Autodesk Inventor part; units mm, degrees
ref_plane "YZ Plane" through (0, 0, 0) normal (1, 0, 0) x (0, 1, 0)
ref_plane "XZ Plane" through (0, 0, 0) normal (0, 1, 0) x (-1, 0, 0)
ref_plane "XY Plane" through (0, 0, 0) normal (0, 0, 1) x (1, 0, 0)
sketch "Sketch1" plane through (0, 0, 0) normal (0, 0, 1) x (1, 0, 0)
  line L0 (0, 0) -> (28.575, 0)
  line L1 (28.575, 0) -> (28.575, 19.05)
  line L2 (28.575, 19.05) -> (0, 19.05)
  line L3 (0, 19.05) -> (0, 0)
  arc A0 (23.8125, 14.2875) -> (23.8125, 7.9375) centre (23.8125, 11.1125) ccw
  arc A1 (4.7625, 7.9375) -> (4.7625, 14.2875) centre (4.7625, 11.1125) ccw
  line L4 (0, 7.9375) -> (4.7625, 7.9375)
  line L5 (0, 14.2875) -> (4.7625, 14.2875)
  line L6 (28.575, 14.2875) -> (23.8125, 14.2875)
  line L7 (28.575, 7.9375) -> (23.8125, 7.9375)
  dimension "d4" = 28.575
  dimension "d5" = 19.05
  dimension "d18" = 7.9375
  dimension "d19" = 4.7625
  dimension "d20" = 7.9375
  dimension "d21" = 4.7625
  dimension "d22" = 6.35
  dimension "d23" = 6.35
  dimension "d24" = 4.7625
  dimension "d25" = 4.7625
  dimension "d26" = 4.7625
  dimension "d27" = 4.7625
extrude "Extrusion1" add sketch "Sketch1" along normal blind 3.175
sketch "Sketch3" plane through (0, 19.05, 0) normal (0, 1, 0) x (1, 0, 0)
  line L0 (0, 0) -> (28.575, 0)
  line L1 (0, 0) -> (28.575, 0)
  line L2 (28.575, 0) -> (28.575, -6.35)
  line L3 (28.575, -6.35) -> (0, -6.35)
  line L4 (0, 0) -> (0, -3.175)
  line L5 (0, 0) -> (0, -22.225)
  circle A0 centre (6.35, -22.225) radius 6.35
  line L6 (28.575, -6.35) -> (11.1411, -26.3925)
  circle A1 centre (6.35, -22.225) radius 3.175
  dimension "d6" = 6.35
  dimension "d8" = 22.225
  dimension "d10" = 28.575
  dimension "d12" = 12.7
  dimension "d13" = 6.35
  dimension "d16" = 6.35
extrude "Extrusion2" add sketch "Sketch3" along normal blind 3.175
fillet "Fillet1" radius 3.175 1 edges at (14.2875, 22.225, 0)
sketch "Sketch4" plane through (0, 0, 0) normal (0, 0, -1) x (-1, 0, 0)
  arc A0 (-23.8125, 7.9375) -> (-23.8125, 14.2875) centre (-23.8125, 11.1125) ccw
  arc A1 (-4.7625, 14.2875) -> (-4.7625, 7.9375) centre (-4.7625, 11.1125) ccw
  line L0 (-28.575, 19.05) -> (0, 19.05)
  line L1 (-28.575, 0) -> (-28.575, 19.05)
  line L2 (0, 0) -> (0, 19.05)
  line L3 (-28.575, 0) -> (-28.575, 19.05)
  line L4 (-28.575, 14.2875) -> (-23.8125, 14.2875)
  line L5 (-28.575, 7.9375) -> (-23.8125, 7.9375)
  line L6 (0, 19.05) -> (0, 0)
  line L7 (0, 14.2875) -> (-4.7625, 14.2875)
  line L8 (0, 7.9375) -> (-4.7625, 7.9375)
  dimension "d28" = 6.35
  dimension "d29" = 6.35
  dimension "d30" = 7.9375
  dimension "d31" = 7.9375
  dimension "d32" = 4.7625
  dimension "d33" = 4.7625
  dimension "d34" = 4.7625
  dimension "d35" = 4.7625
  dimension "d36" = 4.7625
  dimension "d38" = 4.7625
extrude "Extrusion3" cut sketch "Sketch4" against normal through all
fillet "Fillet2" radius 1.5875 2 edges at (28.575, 0, 1.5875) (0, 0, 1.5875)
equation "\"d23\" = d22"
equation "\"d24\" = d21"
equation "\"d26\" = d19"
equation "\"d27\" = d19"
equation "\"d29\" = d28"
equation "\"d31\" = d30"
equation "\"d34\" = d32"
equation "\"d35\" = d32"
equation "\"d36\" = d33"
equation "\"d38\" = d33"
properties part number "LeftAngleBracket-1111-2018" material "Aluminum 6061"
Geometry: final body of the model. Coordinates: model frame, mm. A direction names the side the tool comes from. Give positions to 0.01 mm unless a question says otherwise; leave off trailing zeros. Write each loop counter-clockwise with the first axis right and the second up, starting at its lowest first coordinate (ties: lowest second). Pieces come first, ordered by that corner, then holes.
1. Pin query (flat end, axial travel): P1, Ø3, axis at x = 19.5, y = 5, coming from the +Z side (3 decimals); P2, Ø12.5, axis at x = 17.5, z = 15, coming from the -Y side; P3, Ø2.5, axis at x = 2.5, z = 1.5, coming from the +Y side. Return the tip coordinate at first contact, or that it passes through.
2. Draft query along Y for faces 6 (the flat face through (2, 7.938, 2)), 7 (the flat face through (19.98, 20.62, 16.23)), 8 (the cylindrical face through (7.937, 11.182, 1.565)), 9 (the flat face through (11, 19.05, 13)). Return one class per face: released by +Y, released by -Y, zero draft, split by the parting line, or undercut.
3. Line query: probe 1 along Y at (x, z) = (18, 9.25) (3 decimals); probe 2 along Z at (x, y) = (12, 2) (3 decimals); probe 3 along Z at (x, y) = (6.35, 20.9) (3 decimals). Output: solid intervals per line, ascending.
4. Section query A-A, the plane x = 6.35. Return loops of the section in (y, z) (3 decimals), then the cut area to 3 significant figures.
5. Section query C-C, the plane z = 20. Return loops of the section in (x, y) (3 decimals).
6. Reachability of faces 1 (the flat face through (14, 0, 2)), 2 (the flat face through (11, 22.225, 13)), 3 (the flat face through (2, 14.288, 2)), 4 (the flat face through (26, 14.288, 2)), 5 (the flat face through (14, 10, 3.175)) from +Z, -Z, +X, -X, +Y, -Y: full face, straight path, thin tool, end or side. Return the list, or none.
7. Section query D-D, the plane x = 12.5. Return loops of the section in (y, z) (3 decimals), then the cut area to 3 significant figures.
Computed:
1. P1: stops at z = 3.175
1. P2: stops at y = 19.05
1. P3: stops at y = 22.2
2. face 6: undercut
2. face 7: zero draft
2. face 8: undercut
2. face 9: released by -Y
3. probe 1: y = 19.05 to 22.225
3. probe 2: z = 0 to 3.175
3. probe 3: z = 0.595 to 19.05, 25.4 to 28.575
4. outline: (0, 0) - (8.363, 0) - (8.363, 3.175) - (0, 3.175) - close; (13.862, 0) - (19.05, 0) arc R3.175 ccw to (22.225, 3.175) - (22.225, 19.05) - (19.05, 19.05) - (19.05, 3.175) - (13.862, 3.175) - close; (19.05, 25.4) - (22.225, 25.4) - (22.225, 28.575) - (19.05, 28.575) - close
4. area: 111 mm2
5. outline: (0, 19.05) - (4.085, 19.05) - (4.085, 22.225) - (0, 22.225) - close; (8.615, 19.05) - (16.702, 19.05) - (16.702, 22.225) - (8.615, 22.225) - close
6. face 1: +Z, -Z, +X, -X, -Y
6. face 2: +Z, -Z, +X, -X, +Y
6. face 3: +Z, -Z, -X
6. face 4: +Z, -Z, +X
6. face 5: +Z, +X, -X, -Y
7. outline: (0, 0) - (19.05, 0) arc R3.175 ccw to (22.225, 3.175) - (22.225, 24.83) - (19.05, 24.83) - (19.05, 3.175) - (0, 3.175) - close
7. area: 137 mm2
